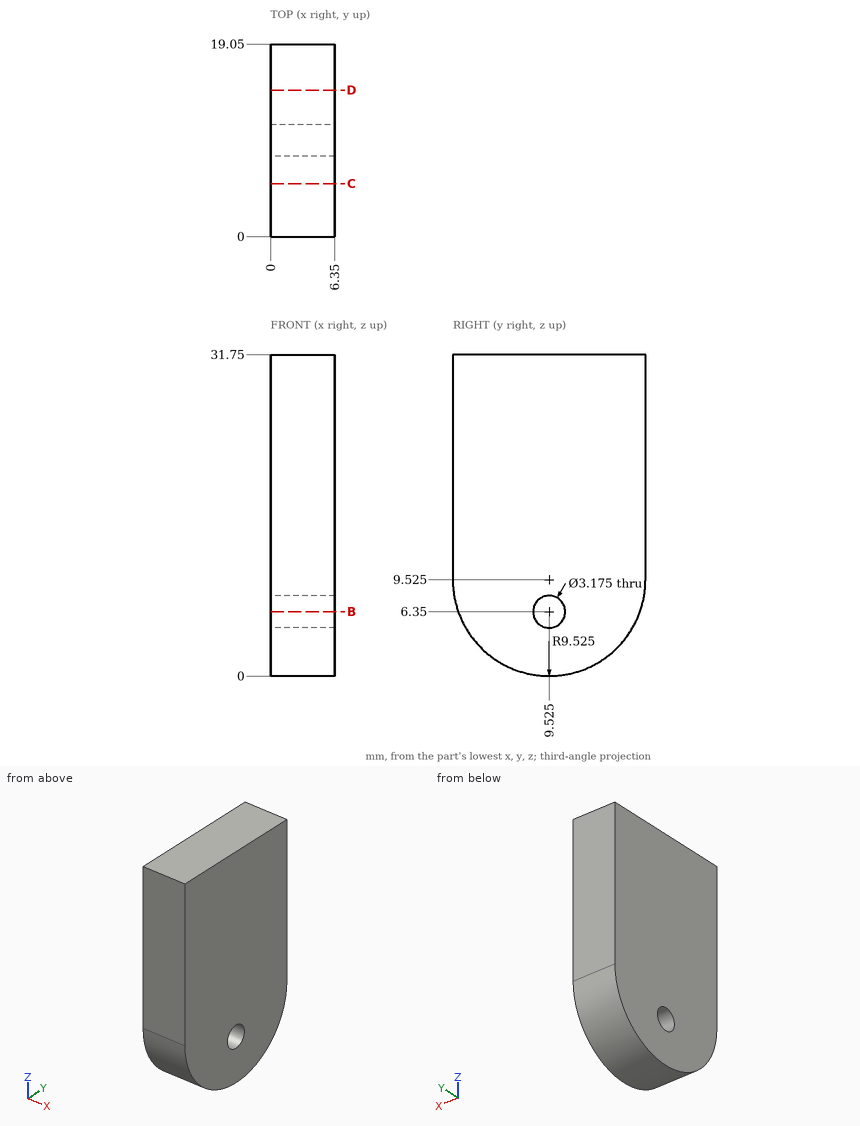
Study the drawing (mm; zero at the part's minimum x, y, z) and answer. Round coordinates to 2 decimals unless told otherwise and drop trailing zeros. Loops run counter-clockwise (first coordinate to the right, second up) from the corner with the lowest first, then second, coordinate; pieces in that order, holes last. Notation, with made-up numbers: (63.5, 5.25) -> (91.5, 5.25) arc R9 ccw to (91.5, 11.25) -> close; hole circle Ø7 at (80, -20.5). An arc over 180 degrees is marked (long way). Use one line per item in the form item = value.
1. Find the intervals of material crossed by probe 1 along Y at (x, z) = (3, 5); probe 2 along Z at (x, y) = (3.25, 9.25); probe 3 along Y at (x, z) = (4.75, 6.5), in increasing order. Write a range as [from, to].
Answer key:
probe_1 = [1.14, 8.69], [10.36, 17.91]
probe_2 = [0, 4.79], [7.91, 31.75]
probe_3 = [0.49, 7.94], [11.11, 18.56]
2. A flat-ended cylindrical pin translates along its axis: pin 1 Ø1.5 at (x, y) = (3, 12.5) entering from -Z. Find the tip coordinate at first contact, or state that the pin passes through.
Answer key:
pin_1 = 0.26
3. The part is cut by section B-B on z = 6.35. Determine the outline of the cut face in (x, y).
Answer key:
outline = (0, 0.54) -> (6.35, 0.54) -> (6.35, 7.94) -> (0, 7.94) -> close; (0, 11.11) -> (6.35, 11.11) -> (6.35, 18.51) -> (0, 18.51) -> close
4. The part is cut by section D-D on y = 14.5. Determine the outline of the cut face in (x, z).
Answer key:
outline = (0, 1.4) -> (6.35, 1.4) -> (6.35, 31.75) -> (0, 31.75) -> close
5. The part is cut by section C-C on y = 5.25. Determine the outline of the cut face in (x, z).
Answer key:
outline = (0, 1.01) -> (6.35, 1.01) -> (6.35, 31.75) -> (0, 31.75) -> close
